CAD build for the part. Positions are in the model's coordinates, mm. A direction names the side the tool comes from. Round coordinates to 2 decimals unless told otherwise and drop trailing zeros. Order: outer loops, then holes, each group sorted by start corner. A loop starts at its lowest first (then second) coordinate and runs counter-clockwise, first axis right, second up. Notation, with made-up numbers: (40.25, 68.5) - (74.25, 68.5) arc R21 ccw to (74.25, 102.5) - close; hole circle Ø2 at (62.5, -1). An arc over 180 degrees is marked (long way). Write item = value, one per line.
from build123d import *

# Parameters (mm, degrees)
BOSS_EXTRUDE1_DEPTH  = 50
SKETCH4_R            = 11
CUT_EXTRUDE1_DEPTH   = 88.099081511
BOSS_EXTRUDE2_DEPTH  = 15
M3_CLEARANCE_HOLE2_D = 3.4
CUT_EXTRUDE2_START   = -6.5
CUT_EXTRUDE2_DEPTH   = 6.5
CUT_EXTRUDE3_START   = -21.5
CUT_EXTRUDE3_DEPTH   = 21.5
FILLET1_R            = 25
FILLET2_R            = 10
CONVERT_SOLID1_START = -21.5
CONVERT_SOLID1_DEPTH = 15
M3_CLEARANCE_HOLE3_D = 3.4


# Read off the part's stored shape, not the designer's step: Convert-Solid1
with BuildPart() as part:
    # Sketch2 → Boss-Extrude1 (new body)
    with BuildSketch(Plane(origin=(0, 0, 0), x_dir=(1, 0, 0), z_dir=(0, 1, 0))):
        with BuildLine():
            Line((0, 0), (-63, 0))
            ThreePointArc((-63, 0), (-66.535533906, 1.464466094), (-68, 5))
            Line((-68, 5), (-68, 21.5))
            Line((-68, 21.5), (-66, 21.5))
            Line((-66, 21.5), (-66, 5))
            ThreePointArc((-66, 5), (-65.121320344, 2.878679656), (-63, 2))
            Line((-63, 2), (0, 2))
            Line((0, 2), (0, 0))
        make_face()
    extrude(amount=BOSS_EXTRUDE1_DEPTH)

    # Sketch4 → Cut-Extrude1 (cut, through all)
    with BuildSketch(Plane.XY):
        with Locations((-25, 25)):
            Circle(SKETCH4_R)
    extrude(amount=-CUT_EXTRUDE1_DEPTH, mode=Mode.SUBTRACT)

    # Sketch3 → Boss-Extrude2 (add)
    with BuildSketch(Plane(origin=(0, 0, -21.5), x_dir=(-1, 0, 0), z_dir=(0, 0, -1))):
        with BuildLine():
            Line((66, 0), (66, -7))
            ThreePointArc((66, -7), (64.828427125, -9.828427125), (62, -11))
            Line((62, -11), (48, -11))
            Line((48, -11), (48, -13))
            Line((48, -13), (63, -13))
            ThreePointArc((63, -13), (66.535533906, -11.535533906), (68, -8))
            Line((68, -8), (68, 0))
            Line((68, 0), (66, 0))
        make_face()
    extrude(amount=-BOSS_EXTRUDE2_DEPTH)

    # M3 Clearance Hole2 (through all)
    with Locations(Plane.XY):
        with Locations((-35.606601718, 14.393398282), (-35.606601718, 35.606601718), (-14.393398282, 35.606601718), (-14.393398282, 14.393398282)):
            Hole(M3_CLEARANCE_HOLE2_D / 2)

    # Sketch8 → Cut-Extrude2 (cut)
    with BuildSketch(Plane.XY.offset(CUT_EXTRUDE2_START)):
        with BuildLine():
            Line((-25, 0), (-68, 0))
            Line((-68, 0), (-68, 17.5))
            Line((-68, 17.5), (-48.848480035, 17.5))
            ThreePointArc((-48.848480035, 17.5), (-39.790199458, 4.844355629), (-25, 0))
        make_face()
    extrude(amount=CUT_EXTRUDE2_DEPTH, mode=Mode.SUBTRACT)

    # Sketch9 → Cut-Extrude3 (cut)
    with BuildSketch(Plane.XY.offset(CUT_EXTRUDE3_START)):
        with BuildLine():
            Line((-25, 50), (-68, 50))
            Line((-68, 50), (-68, 32.5))
            Line((-68, 32.5), (-48.848480035, 32.5))
            ThreePointArc((-48.848480035, 32.5), (-39.790199458, 45.155644371), (-25, 50))
        make_face()
    extrude(amount=CUT_EXTRUDE3_DEPTH, mode=Mode.SUBTRACT)

    # Fillet1
    fillet1_edges = [part.edges().sort_by_distance(p)[0] for p in [
        (0, 0, -1),
        (0, 50, -1),
    ]]
    fillet(fillet1_edges, radius=FILLET1_R - 0.0001)  # a hair under: the kernel refuses the full size

    # Fillet2
    fillet2_edges = [part.edges().sort_by_distance(p)[0] for p in [
        (-48.848480035, 32.5, -1),
        (-48.848480035, 17.5, -1),
    ]]
    fillet(fillet2_edges, radius=FILLET2_R)

    # Convert-Solid1 outline → Convert-Solid1 (cut)
    with BuildSketch(Plane.XY.offset(CONVERT_SOLID1_START)):
        with BuildLine():
            Line((-63, -13), (-62, -13))
            ThreePointArc((-62, -13), (-66.242640687, -11.242640687), (-68, -7))
            Line((-68, -7), (-68, -8))
            ThreePointArc((-68, -8), (-66.535533906, -11.535533906), (-63, -13))
        make_face()
    extrude(amount=CONVERT_SOLID1_DEPTH, mode=Mode.SUBTRACT)

    # M3 Clearance Hole3 (through all)
    with Locations(Plane(origin=(0, -11, 0), x_dir=(1, 0, 0), z_dir=(0, 1, 0))):
        with Locations((-54, 10), (-54, 18)):
            Hole(M3_CLEARANCE_HOLE3_D / 2)


solid = part.part
(1) Band-saw the part on D-D on y = 19. List the corners of the cut face in (x, z).
Solved:
outline = (-68, -21.5) - (-66, -21.5) - (-66, -5) arc R3 cw to (-63, -2) - (-34.22, -2) - (-34.22, 0) - (-63, 0) arc R5 ccw to (-68, -5) - close; (-15.78, -2) - (-0.73, -2) - (-0.73, 0) - (-15.78, 0) - close
(2) Band-saw the part on C-C on x = -15. List the corners of the cut face in (y, z).
Solved:
outline = (2.09, -2) - (12.81, -2) - (12.81, 0) - (2.09, 0) - close; (15.98, -2) - (20.42, -2) - (20.42, 0) - (15.98, 0) - close; (29.58, -2) - (34.02, -2) - (34.02, 0) - (29.58, 0) - close; (37.19, -2) - (47.91, -2) - (47.91, 0) - (37.19, 0) - close
(3) Band-saw the part on A-A on z = -10. List the corners of the cut face in (x, y), plus the area to 3 significant figures.
Solved:
outline = (-68, -7) arc R6 ccw to (-62, -13) - (-55.7, -13) - (-55.7, -11) - (-62, -11) arc R4 cw to (-66, -7) - (-66, 32.5) - (-68, 32.5) - close; (-52.3, -13) - (-48, -13) - (-48, -11) - (-52.3, -11) - close
area = 116 mm²
(4) Probe line 1 along Z through (x, y) = (-54, -12); line 2 along Y through (x, z) = (-25, -0.4); line 3 along Z through (x, y) = (-15, 6.5). List the from-to ranges inside material, lowest first.
Solved:
line_1 = -21.5 to -19.7, -16.3 to -11.7, -8.3 to -6.5
line_2 = 0 to 14, 36 to 50
line_3 = -2 to 0
(5) Pull direction Y, two halves, no side cores. Call faces 4 (the cylindrical face through (-37.658, 3.442, -1.014)), 5 (the cylindrical face through (-36.391, 12.885, -1.014)), 6 (the cylindrical face through (-13.14, 36.756, -1.014)), 7 (the flat face through (-38, 25, 0)): released by +Y, released by -Y, zero draft, split by the parting line, or undercut.
Solved:
face_4 = released by -Y
face_5 = undercut
face_6 = undercut
face_7 = zero draft
(6) Tool access for faces 1 (the flat face through (-66.4, 32.5, -8.4)), 2 (the flat face through (-55, -11, -14)), 3 (the flat face through (-66, 13, -13)): list every direction of +Z, -Z, +X, -X, +Y, -Y with a clear straight run to the whole face (end or side of a thin tool).
Solved:
face_1 = +Z, -Z, -X, +Y
face_2 = +Z, -Z, +X, +Y
face_3 = -Z, +X, +Y
(7) Drop flat-ended pins along their axis: pin 1 (8 mm diameter, centred on y = 12, z = -11.5, fed in from +X); pin 2 (4 mm diameter, centred on x = -54.5, z = -11.5, fed in from +Y); pin 3 (6 mm diameter, centred on x = -50, y = 13, fed in from +Z); pin 4 (4 mm diameter, centred on x = -9.5, y = 0.5, fed in from +Z). Give the stop position or say it passes through.
Solved:
pin_1 = -66
pin_2 = -11
pin_3 = 0
pin_4 = through
(8) Band-saw the part on B-B on x = -57. List the corners of the cut face in (y, z), plus the area to 3 significant figures.
Solved:
outline = (-13, -21.5) - (-11, -21.5) - (-11, -6.5) - (-13, -6.5) - close; (17.5, -2) - (32.5, -2) - (32.5, 0) - (17.5, 0) - close
area = 60.0 mm²
